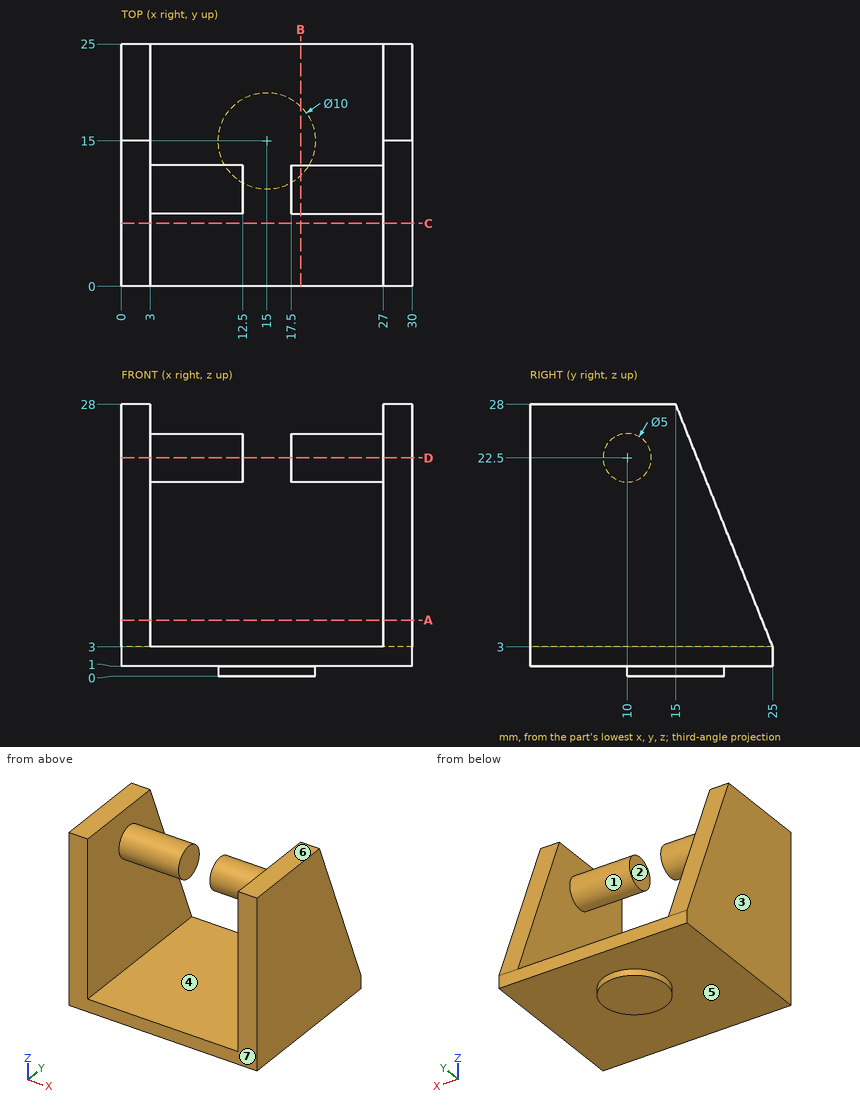
Part print with two shaded views. Sizes in mm from the minimum x, y, z corner. A direction names the side the tool comes from. Coordinates: 2 decimals unless noted, no trailing zeros. Loops run counter-clockwise (first coordinate to the right, second up) from the corner with the lowest first, then second, coordinate; pieces in that order, holes last. Notation, with made-up numbers: M 82,-10 L 111,-10 A29 cw 111,11 Z; hole C 54,23.25 d3. An arc over 180 degrees is marked long. Use CSV: the item, a comma, the result in double quotes. Start each with the question number.
1. Flat gauge pins, fed straight in: pin 1 (2 mm diameter, centred on x = 17, y = 14, fed in from -Z); pin 2 (1 mm diameter, centred on x = 10.5, y = 15, fed in from +Z). Where does each tip first touch, or does it go through?
2. Band-saw the part on A-A, the plane z = 5.75. List the corners of the cut face in (x, y).
3. Probe probe 1 along X at (y, z) = (21.25, 4.25); probe 2 along Z at (x, y) = (8, 17.5); probe 3 along Z at (x, y) = (19, 13.5). List the from-to ranges inside material, lowest first. Write a range as [from, to].
4. Band-saw the part on B-B, the plane x = 18.5. List the corners of the cut face in (y, z), then the cut area to 3 significant figures.
5. Tool access for the marked faces 1, 2 and 3: list every direction of +Z, -Z, +X, -X, +Y, -Y with a clear straight run to the whole face (end or side of a thin tool).
6. Two-plate mould, pull along Z, no slides. Class the marked faces 4, 5, 6 and 7: pulls with the +Z half, pulls with the -Z half, needs draft (parallel to the pull), parting line crosses it, or undercut.
7. Band-saw the part on C-C, the plane y = 6.5. List the corners of the cut face in (x, z), then the cut area to 3 significant figures.
8. Band-saw the part on D-D, the plane z = 22.5. List the corners of the cut face in (x, y).
Entries:
1,pin 1,"stops at z = 0"
1,pin 2,"stops at z = 3"
2,outline,"M 0,0 L 3,0 L 3,23.9 L 0,23.9 Z; M 27,0 L 30,0 L 30,23.9 L 27,23.9 Z"
3,probe 1,"x = [0, 3], [27, 30]"
3,probe 2,"z = [1, 3]"
3,probe 3,"z = [0, 3]"
4,outline,"M 0,1 L 11.43,1 L 11.43,0 L 18.57,0 L 18.57,1 L 25,1 L 25,3 L 0,3 Z; C 10,22.5 d5"
4,area,"76.8 mm2"
5,face 1,"none"
5,face 2,"+Z, +Y, -Y"
5,face 3,"+Z, -Z, -X, +Y, -Y"
6,face 4,"undercut"
6,face 5,"pulls with the -Z half"
6,face 6,"pulls with the +Z half"
6,face 7,"needs draft"
7,outline,"M 0,1 L 30,1 L 30,28 L 27,28 L 27,3 L 3,3 L 3,28 L 0,28 Z"
7,area,"210 mm2"
8,outline,"M 0,0 L 3,0 L 3,7.5 L 12.5,7.5 L 12.5,12.5 L 3,12.5 L 3,17.2 L 0,17.2 Z; M 17.5,7.5 L 27,7.5 L 27,0 L 30,0 L 30,17.2 L 27,17.2 L 27,12.5 L 17.5,12.5 Z"
